Build history of the part. All positions in model axes, mm. A direction names the side the tool comes from. Give positions to 0.01 mm unless a question says otherwise; leave off trailing zeros. Write each loop counter-clockwise with the first axis right and the second up, starting at its lowest first coordinate (ties: lowest second). Pieces come first, ordered by that corner, then holes. Notation, with made-up numbers: (-19, -25.75) -> (29, -25.75) arc R21 cw to (29, 1.25) -> close; hole circle Ø7 at (-37, 4.25). An arc over 180 degrees is marked (long way). One line per question, with ' | ' between items. Start each with the question number.
(1) Tool access for faces 1 (the flat face through (21, -1, 23)), 2 (the flat face through (-10, -9, 42)), 3 (the flat face through (6.36, -9.25, 22.82)), 4 (the flat face through (10, -9, 3)): list every direction of +Z, -Z, +X, -X, +Y, -Y with a clear straight run to the whole face (end or side of a thin tool).
(2) Drill centre lines: probe 1 along Z at (x, y) = (16, 11); probe 2 along X at (y, z) = (0, 2.7); probe 3 along Z at (x, y) = (12.5, 3). Where is each one in solid material? Low to high. Write a range as from..to.
(3) Band-saw the part on B-B, the plane z = 7.5. Give the cut face in (x, y), and give its area (3 significant figures).
(4) Band-saw the part on C-C, the plane x = -16. Give the cut face in (y, z).
(5) Band-saw the part on D-D, the plane x = -6. Give the cut face in (y, z).
(6) Pull direction Z, two halves, no side cores. Call faces 5 (the cylindrical face through (-18, 13, 39)), 6 (the flat face through (-22.5, 16, 23)), 7 (the flat face through (3, 13, 2)), 8 (the flat face through (-16, 6, 37)): released by +Z, released by -Z, zero draft, split by the parting line, or undercut.
(7) Pin check, flat tips, straight feed: P1, Ø4, axis at y = -1.5, z = 38, coming from the -X side; P2, Ø1, axis at x = -2.5, y = 11.5, coming from the +Z side; P3, Ø2, axis at x = -4, z = 18, coming from the +Y side; P4, Ø3, axis at x = -8.5, z = 12.5, coming from the +Y side. Stop position of each tip, or through.
from build123d import *

# Parameters (mm, degrees)
RESSALTO_EXTRUS_O1_DEPTH = 45
ESBO_O3_R                = 14
CORTE_EXTRUS_O2_DEPTH    = 3
ESBO_O4_R                = 8.659932388
ESBO_O4_R_2              = 8
RESSALTO_EXTRUS_O2_DEPTH = 1
CORTE_EXTRUS_O3_DEPTH    = 1
ESBO_O6_R                = 0.581806569
RESSALTO_EXTRUS_O3_DEPTH = 1
ESBO_O8_W                = 66.682798833
ESBO_O8_H                = 46.433556561
CORTE_EXTRUS_O5_DEPTH    = 23.5
ESBO_O9_R                = 2.5
CORTE_EXTRUS_O6_DEPTH    = 14


with BuildPart() as part:
    # Esboço1 → Ressalto-extrusão1 (new body)
    with BuildSketch(Plane.XY):
        with BuildLine():
            Line((-22.5, 20), (-22.5, 11))
            Line((-22.5, 11), (-21, 9.864062641))
            Line((-21, 9.864062641), (-21, -11.8))
            Line((-21, -11.8), (-8.5, -11.8))
            Line((-8.5, -11.8), (-4.27343132, -6.762971592))
            ThreePointArc((-4.27343132, -6.762971592), (0, 8), (4.27343132, -6.762971592))
            Line((4.27343132, -6.762971592), (8.5, -11.8))
            Line((8.5, -11.8), (21, -11.8))
            Line((21, -11.8), (21, 9.864062641))
            Line((21, 9.864062641), (22.5, 11))
            Line((22.5, 11), (22.5, 20))
            Line((22.5, 20), (9.5, 20))
            Line((9.5, 20), (8.5, 19.2))
            Line((8.5, 19.2), (-8.5, 19.2))
            Line((-8.5, 19.2), (-9.5, 20))
            Line((-9.5, 20), (-22.5, 20))
        make_face()
    extrude(amount=RESSALTO_EXTRUS_O1_DEPTH)

    # Esboço3 → Corte-extrusão2 (cut)
    with BuildSketch(Plane(origin=(0, 0, 0), x_dir=(-1, 0, 0), z_dir=(0, 0, -1))):
        Circle(ESBO_O3_R)
    extrude(amount=-CORTE_EXTRUS_O2_DEPTH, mode=Mode.SUBTRACT)

    # Esboço4 → Ressalto-extrusão2 (add)
    with BuildSketch(Plane(origin=(0, 0, 3), x_dir=(-1, 0, 0), z_dir=(0, 0, -1))):
        Circle(ESBO_O4_R)
        Circle(ESBO_O4_R_2, mode=Mode.SUBTRACT)
    extrude(amount=RESSALTO_EXTRUS_O2_DEPTH)

    # Esboço5 → Corte-extrusão3 (cut)
    with BuildSketch(Plane(origin=(0, 0, 3), x_dir=(-1, 0, 0), z_dir=(0, 0, -1))):
        Polygon((-8.150170401, -11.383089319), (-4.701200585, -7.27276715), (-4.703249192, -5.654958468), (3.343697917, -5.654958468), (4.701200585, -7.27276715), (8.150170401, -11.383089319), (0.388307104, -10.144815057), align=None)
    extrude(amount=CORTE_EXTRUS_O3_DEPTH, mode=Mode.SUBTRACT)

    # Esboço6 → Ressalto-extrusão3 (add)
    with BuildSketch(Plane(origin=(0, 0, 3), x_dir=(-1, 0, 0), z_dir=(0, 0, -1))):
        with BuildLine():
            Line((-8.96541648, -9.883119832), (-9.879437481, -10.890700362))
            ThreePointArc((-9.879437481, -10.890700362), (0, 14.704102805), (9.879437481, -10.890700362))
            Line((9.879437481, -10.890700362), (8.96541648, -9.883119832))
            ThreePointArc((8.96541648, -9.883119832), (8.661852403, -8.191590578), (10.346023957, -7.849554692))
            ThreePointArc((10.346023957, -7.849554692), (0, 12.986751733), (-10.346023957, -7.849554692))
            ThreePointArc((-10.346023957, -7.849554692), (-8.661852403, -8.191590578), (-8.96541648, -9.883119832))
        make_face()
        with Locations((-9.678899136, -8.882073659)):
            Circle(ESBO_O6_R, mode=Mode.SUBTRACT)
        with Locations((9.678899136, -8.882073659)):
            Circle(ESBO_O6_R, mode=Mode.SUBTRACT)
    extrude(amount=RESSALTO_EXTRUS_O3_DEPTH)

    # Esboço8 → Corte-extrusão5 (cut, through all)
    with BuildSketch(Plane.XY.offset(22.5)):
        with Locations((0.496680915, 3.185740871)):
            Rectangle(ESBO_O8_W, ESBO_O8_H)
    extrude(amount=CORTE_EXTRUS_O5_DEPTH, mode=Mode.SUBTRACT)

    # Espelhar14: part across plane


with BuildPart() as part_1:
    add(part.part)
    add(part.part.mirror(Plane.XY.offset(22.5)))

    # Esboço9 → Corte-extrusão6 (cut)
    with BuildSketch(Plane(origin=(0, 20, 0), x_dir=(1, 0, 0), z_dir=(0, 1, 0))):
        with Locations((-16, -7.5)):
            Circle(ESBO_O9_R)
        with Locations((16, -7.5)):
            Circle(ESBO_O9_R)
        with Locations((16, -37.5)):
            Circle(ESBO_O9_R)
        with Locations((-16, -37.5)):
            Circle(ESBO_O9_R)
    extrude(amount=-CORTE_EXTRUS_O6_DEPTH, mode=Mode.SUBTRACT)


solid = part_1.part
Results:
1) face 1: +Z, -Z, +X, -Y | face 2: +Z | face 3: +Z, -Z, -Y | face 4: -Z
2) probe 1: z = 0..5, 10..35, 40..45 | probe 2: x = -21..-12.99, -8.66..-8, 8..8.66, 12.99..21 | probe 3: z = 3..42
3) outline: (-22.5, 11) -> (-21, 9.86) -> (-21, -11.8) -> (-8.5, -11.8) -> (-4.27, -6.76) arc R8 cw (long way) to (4.27, -6.76) -> (8.5, -11.8) -> (21, -11.8) -> (21, 9.86) -> (22.5, 11) -> (22.5, 20) -> (18.5, 20) -> (18.5, 6) -> (13.5, 6) -> (13.5, 20) -> (9.5, 20) -> (8.5, 19.2) -> (-8.5, 19.2) -> (-9.5, 20) -> (-13.5, 20) -> (-13.5, 6) -> (-18.5, 6) -> (-18.5, 20) -> (-22.5, 20) -> close | area: 952 mm²
4) outline: (-11.8, 0) -> (20, 0) -> (20, 5) -> (6, 5) -> (6, 10) -> (20, 10) -> (20, 35) -> (6, 35) -> (6, 40) -> (20, 40) -> (20, 45) -> (-11.8, 45) -> close
5) outline: (-8.82, 3) -> (-6.24, 3) -> (-6.24, 2) -> (-5.29, 2) -> (-5.29, 43) -> (-6.24, 43) -> (-6.24, 42) -> (-8.82, 42) -> close; (5.29, 2) -> (6.24, 2) -> (6.24, 3) -> (11.52, 3) -> (11.52, 2) -> (12.65, 2) -> (12.65, 0) -> (19.2, 0) -> (19.2, 45) -> (12.65, 45) -> (12.65, 43) -> (11.52, 43) -> (11.52, 42) -> (6.24, 42) -> (6.24, 43) -> (5.29, 43) -> close
6) face 5: undercut | face 6: zero draft | face 7: released by -Z | face 8: undercut
7) P1: stops at x = -21 | P2: stops at z = 42 | P3: stops at y = 19.2 | P4: stops at y = 20
